Geometry: final body of the model. Coordinates: model frame, mm. Give positions to 0.01 mm unless a question says otherwise; leave off trailing zeros. Write each loop counter-clockwise with the first axis right and the second up, starting at its lowest first coordinate (ties: lowest second). Pieces come first, ordered by that corner, then holes.
```python
from build123d import *

# Parameters (mm, degrees)
F0_R     = 10.16
F1_DEPTH = 15.24
F2_R     = 2.54
F3_R     = 1.27
F4_DEPTH = 35.56


with BuildPart() as f1:
    # F0 (on Top) → F1 (new body)
    with BuildSketch(Plane.XY):
        Circle(F0_R)
    extrude(amount=F1_DEPTH)

    # F2
    f2_edges = [f1.edges().sort_by_distance(p)[0] for p in [
        (-10.16, 0, 15.24),
        (-10.16, 0, 0),
    ]]
    fillet(f2_edges, radius=F2_R)

    # F3 (on face) → F4 (join)
    with BuildSketch(Plane.XY.offset(15.24)):
        Circle(F3_R)
    extrude(amount=F4_DEPTH)


solid = f1.part
```
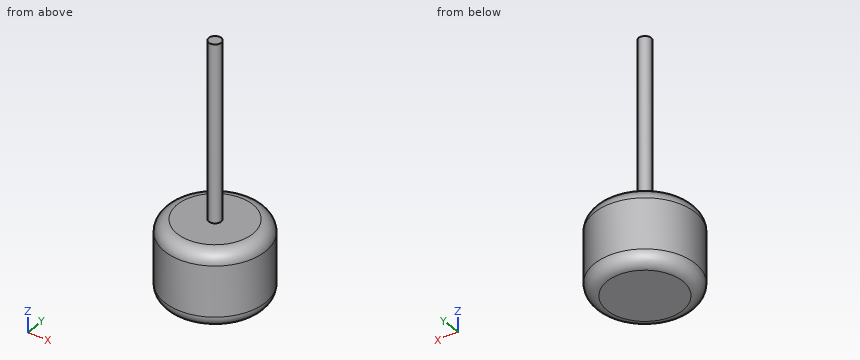
Item 1: Line query: L1, parallel to Z at x = -4, y = 2.5; L2, parallel to X at y = -2, z = 7.5; L3, parallel to X at y = 1, z = 3.5. Output: solid intervals per line, ascending.
Found:
L1: z = 0 to 15.24
L2: x = -9.96 to 9.96
L3: x = -10.11 to 10.11
Item 2: Pin query (flat end, axial travel): pin 1 Ø1.5 at (x, y) = (4, 8) entering from -Z; pin 2 Ø4 at (x, z) = (1.5, 31) entering from +Y; pin 3 Ø5 at (x, z) = (-3, 41) entering from -Y. Return the tip coordinate at first contact, or that it passes through.
Found:
pin 1: stops at z = 0.07
pin 2: stops at y = 1.27
pin 3: stops at y = -1.17
Item 3: Section D-D, the plane z = 5.5. Return the cut outline in (x, y).
Found:
outline: circle Ø20.32 at (0, 0)
Item 4: Section C-C, the plane z = 47.5. Return the cut outline in (x, y).
Found:
outline: circle Ø2.54 at (0, 0)
Item 5: Section A-A, the plane y = 0. Return the cut outline in (x, z).
Found:
outline: (-10.16, 2.54) arc R2.54 ccw to (-7.62, 0) - (7.62, 0) arc R2.54 ccw to (10.16, 2.54) - (10.16, 12.7) arc R2.54 ccw to (7.62, 15.24) - (1.27, 15.24) - (1.27, 50.8) - (-1.27, 50.8) - (-1.27, 15.24) - (-7.62, 15.24) arc R2.54 ccw to (-10.16, 12.7) - close
